from build123d import *

# Parameters (mm, degrees)
F0_W      = 68
F0_H      = 31.5
F1_DEPTH  = 21
F2_W      = 39
F2_H      = 31.5
F3_DEPTH  = 11
F4_R      = 6
F5_DEPTH  = 2
F6_R      = 3
F7_DEPTH  = 34.001
F9_DEPTH  = 10
F11_DEPTH = 31.501
F12_W     = 39
F12_H     = 2
F13_DEPTH = 3
F14_R     = 2.5
F15_DEPTH = 34.001
F17_DEPTH = 25.001
F18_R     = 2
F19_R     = 1.99999


# Not quite as in the source:
# - a fillet or chamfer is up to 0.001 mm smaller than in the source, because OpenCascade refuses the exact size


with BuildPart() as f1:
    # F0 (on Top) → F1 (new body)
    with BuildSketch(Plane.XY):
        Rectangle(F0_W, F0_H)
    extrude(amount=-F1_DEPTH)

    # F2 (on face) → F3 (join)
    with BuildSketch(Plane(origin=(0, 0, -21), x_dir=(1, 0, 0), z_dir=(0, 0, -1))):
        Rectangle(F2_W, F2_H)
    extrude(amount=F3_DEPTH)

    # F4 (on face) → F5 (join)
    with BuildSketch(Plane.XY):
        with Locations((-26, 0)):
            Circle(F4_R)
        with Locations((26, 0)):
            Circle(F4_R)
    extrude(amount=F5_DEPTH)

    # F6 (on face) → F7 (cut, through all)
    with BuildSketch(Plane.XY.offset(2)):
        with Locations((-26, 0)):
            Circle(F6_R)
        with Locations((26, 0)):
            Circle(F6_R)
    extrude(amount=-F7_DEPTH, mode=Mode.SUBTRACT)

    # F8 (on face) → F9 (cut)
    with BuildSketch(Plane(origin=(0, 0, -21), x_dir=(1, 0, 0), z_dir=(0, 0, -1))):
        Polygon((-26, 5.1961524227), (-30.5, 2.5980762114), (-30.5, -2.5980762114), (-26, -5.1961524227), (-21.5, -2.5980762114), (-21.5, 2.5980762114), align=None)
        Polygon((26, -5.1961524227), (30.5, -2.5980762114), (30.5, 2.5980762114), (26, 5.1961524227), (21.5, 2.5980762114), (21.5, -2.5980762114), align=None)
    extrude(amount=-F9_DEPTH, mode=Mode.SUBTRACT)

    # F10 (on face) → F11 (cut, through all)
    with BuildSketch(Plane.XZ.offset(15.75)):
        with BuildLine():
            Line((4.5, -23), (4.5, -16.3935963108))
            ThreePointArc((4.5, -16.3935963108), (13.5185058346, -10.307764064), (17, 0))
            Line((17, 0), (-17, 0))
            ThreePointArc((-17, 0), (-13.5185058346, -10.307764064), (-4.5, -16.3935963108))
            Line((-4.5, -16.3935963108), (-4.5, -23))
            Line((-4.5, -23), (4.5, -23))
        make_face()
    extrude(amount=-F11_DEPTH, mode=Mode.SUBTRACT)

    # F12 (on face) → F13 (join)
    with BuildSketch(Plane(origin=(0, 0, -32), x_dir=(1, 0, 0), z_dir=(0, 0, -1))):
        with Locations((0, 14.75)):
            Rectangle(F12_W, F12_H)
    extrude(amount=F13_DEPTH)

    # F14 (on face) → F15 (cut, through all)
    with BuildSketch(Plane(origin=(0, 0, -32), x_dir=(1, 0, 0), z_dir=(0, 0, -1))):
        with Locations((-6.5, 3.7527767497)):
            Circle(F14_R)
        with Locations((6.5, 3.7527767497)):
            Circle(F14_R)
        with Locations((0, -7.5055534995)):
            Circle(F14_R)
    extrude(amount=-F15_DEPTH, mode=Mode.SUBTRACT)

    # F16 (on face) → F17 (cut, through all)
    with BuildSketch(Plane.XY.offset(-23)):
        with BuildLine():
            ThreePointArc((-6.5, 1.7472232503), (-12, -3.7527767497), (-6.5, -9.2527767497))
            Line((-6.5, -9.2527767497), (6.5, -9.2527767497))
            ThreePointArc((6.5, -9.2527767497), (12, -3.7527767497), (6.5, 1.7472232503))
            Line((6.5, 1.7472232503), (-6.5, 1.7472232503))
        make_face()
    extrude(amount=F17_DEPTH, mode=Mode.SUBTRACT)

    # F18
    f18_edges = [f1.edges().sort_by_distance(p)[0] for p in [
        (-34, -15.75, -10.5),
        (34, -15.75, -10.5),
        (34, 15.75, -10.5),
        (-34, 15.75, -10.5),
    ]]
    fillet(f18_edges, radius=F18_R)

    # F19 (radius 2 in the source; OpenCascade refuses exactly that, so slightly less here)
    f19_edges = [f1.edges().sort_by_distance(p)[0] for p in [
        (-19.5, 0, -21),
        (19.5, 0, -21),
    ]]
    fillet(f19_edges, radius=F19_R)


solid = f1.part
Geometry: final body of the model. Coordinates: model frame, mm. A direction names the side the tool comes from. Round coordinates to 2 decimals unless told otherwise and drop trailing zeros. Loops run counter-clockwise (first coordinate to the right, second up) from the corner with the lowest first, then second, coordinate; pieces in that order, holes last. Notation, with made-up numbers: (-16, 88.25) - (10, 88.25) arc R15 cw to (10, 104.25) - close; hole circle Ø7 at (-19.75, -24.75). An arc over 180 degrees is marked (long way). Write each question's results on one line, items separated by ' | '. Start each with the question number.
1) Cut plane B-B on x = 0. Return loops of the section in (y, z), then the cut area to 4 significant figures.
2) Access query for faces 1 (the face through (27, 3, 2)), 2 (the face through (29, 4, -21)), 3 (the face through (-29, 1, -11)), 4 (the face through (12, -3.9, -18.8)), 5 (the face through (-13.6, -0.2, -10.2)). Directions: +Z, -Z, +X, -X, +Y, -Y. A direction counts if a zero-diameter tool reaches every point of the face in a straight line with its end or side. Return the directions, or none.
3) Cut plane D-D on z = -13. Return loops of the section in (x, y).
4) Cut plane C-C on y = -12. Return loops of the section in (x, z).
5) Cut plane A-A on z = -19. Count the separate pieces of the cut face and the enclosed holes in it, then the cut area to 3 significant figures.
6) First-contact query: P1, Ø5, axis at x = 15.5, y = -8.5, coming from the +Z side; P2, Ø6, axis at y = -7.5, z = -29, coming from the +X side; P3, Ø4, axis at x = -29.5, y = 6.5, coming from the -Z side. Flat tips, straight axial feed; report the tip coordinate or a pass-through.
7) Mould query, pull axis X, two halves, no side actions, for faces 6 (the face through (-33.43, -15.15, -10.65)), 7 (the face through (0, 1, -32)), 8 (the face through (6, 1.747, -19)), 9 (the face through (19.5, 0, -28)). Classes: released by +X, released by -X, zero draft, split by the parting line, or undercut.
8) Line query: probe 1 along Y at (x, z) = (-6.5, -30); probe 2 along Y at (x, z) = (-26, -4); probe 3 along X at (y, z) = (5.5, -17). Output: solid intervals per line, ascending. Write a range as [from, to].
Verdict:
1) outline: (-15.75, -35) - (-13.75, -35) - (-13.75, -32) - (5.01, -32) - (5.01, -23) - (-15.75, -23) - close; (10.01, -32) - (15.75, -32) - (15.75, -23) - (10.01, -23) - close | area: 244.5 mm2
2) face 1: +Z, +X, -X, +Y, -Y | face 2: -Z, +X, +Y, -Y | face 3: -Z | face 4: +Z | face 5: +Z, +Y, -Y
3) outline: (-34, -13.75) arc R2 ccw to (-32, -15.75) - (-10.95, -15.75) - (-10.95, -6.98) arc R5.5 cw to (-10.95, -0.53) - (-10.95, 15.75) - (-32, 15.75) arc R2 ccw to (-34, 13.75) - close; (10.95, -15.75) - (32, -15.75) arc R2 ccw to (34, -13.75) - (34, 13.75) arc R2 ccw to (32, 15.75) - (10.95, 15.75) - (10.95, -0.53) arc R5.5 cw to (10.95, -6.98) - close; hole (-30.5, -2.6) - (-26, -5.2) - (-21.5, -2.6) - (-21.5, 2.6) - (-26, 5.2) - (-30.5, 2.6) - close; hole (21.5, -2.6) - (26, -5.2) - (30.5, -2.6) - (30.5, 2.6) - (26, 5.2) - (21.5, 2.6) - close
4) outline: (-34, -21) - (-21.5, -21) arc R2 cw to (-19.5, -23) - (-19.5, -32) - (19.5, -32) - (19.5, -23) arc R2 cw to (21.5, -21) - (34, -21) - (34, 0) - (17, 0) arc R17 cw to (4.5, -16.39) - (4.5, -23) - (-4.5, -23) - (-4.5, -16.39) arc R17 cw to (-17, 0) - (-34, 0) - close
5) separate pieces: 2 | enclosed holes: 2 | area: 1,580 mm2
6) P1: stops at z = 0 | P2: stops at x = 19.5 | P3: stops at z = -21
7) face 6: released by -X | face 7: zero draft | face 8: undercut | face 9: released by +X
8) probe 1: y = [-15.75, -6.25], [-1.25, 15.75] | probe 2: y = [-15.75, -3], [3, 15.75] | probe 3: x = [-34, -4.5], [4.5, 34]
